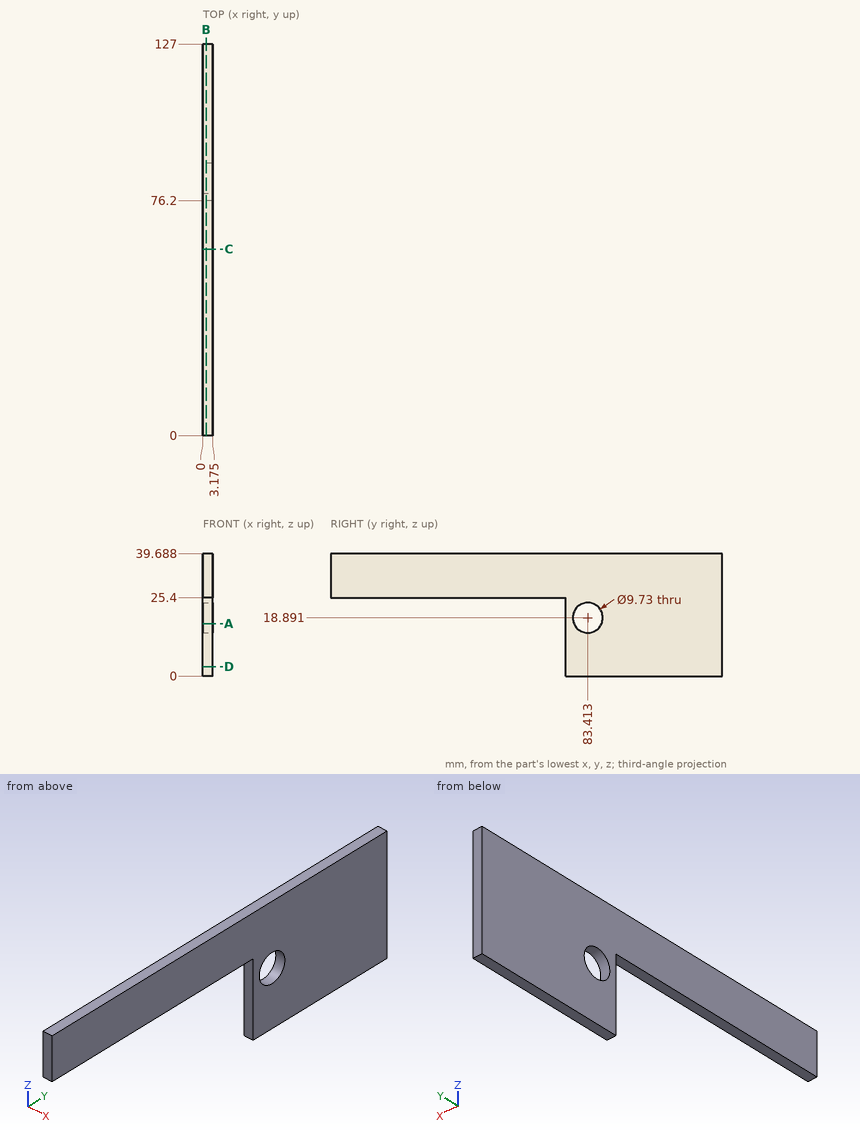
Here's the drawing with two shaded views (mm, measured from the low corner). I have some questions. Coordinates: 2 decimals unless noted, no trailing zeros. Loops run counter-clockwise (first coordinate to the right, second up) from the corner with the lowest first, then second, coordinate; pieces in that order, holes last. Notation, with made-up numbers: (22.25, -7.75) -> (77.25, -7.75) arc R17 cw to (77.25, 4.25) -> close; hole circle Ø7 at (56, 21). An arc over 180 degrees is marked (long way). Answer in a Markdown table with one row per item.
(1) Imagine slicing it at A-A (z = 17). List the corners of the cut face in (x, y) for me (1 decimal), plus the area to 3 significant figures.
Results found:
| item | result |
|---|---|
| outline | (0, 76.2) -> (3.2, 76.2) -> (3.2, 78.9) -> (0, 78.9) -> close; (0, 87.9) -> (3.2, 87.9) -> (3.2, 127) -> (0, 127) -> close |
| area | 133 mm^2 |
(2) Imagine slicing it at C-C (y = 60.5). List the corners of the cut face in (x, z) for me (1 decimal).
Results found:
| item | result |
|---|---|
| outline | (0, 25.4) -> (3.2, 25.4) -> (3.2, 39.7) -> (0, 39.7) -> close |
(3) Imagine slicing it at D-D (z = 3). List the corners of the cut face in (x, y) for me (1 decimal), plus the area to 3 significant figures.
Results found:
| item | result |
|---|---|
| outline | (0, 76.2) -> (3.2, 76.2) -> (3.2, 127) -> (0, 127) -> close |
| area | 161 mm^2 |
(4) If I drill on probe 1 along Y at (x, z) = (2.8, 15.5) (1 decimal); probe 2 along Z at (x, y) = (1, 66.5); probe 3 along Y at (x, z) = (0.9, 9), over which ranges is the centre line in solid material (lowest first)?
Results found:
| item | result |
|---|---|
| probe 1 | y = 76.2 to 79.9, 86.9 to 127 |
| probe 2 | z = 25.4 to 39.69 |
| probe 3 | y = 76.2 to 127 |
(5) Imagine slicing it at B-B (x = 1.1). List the corners of the cut face in (y, z) for me (1 decimal), plus the area to 3 significant figures.
Results found:
| item | result |
|---|---|
| outline | (0, 25.4) -> (76.2, 25.4) -> (76.2, 0) -> (127, 0) -> (127, 39.7) -> (0, 39.7) -> close; hole circle Ø9.7 at (83.4, 18.9) |
| area | 3,030 mm^2 |
(6) Will this pin go through, and if not, where does the flat tip stop? pin 1 Ø1 at (x, y) = (1.5, 35) entering from -Z.
Results found:
| item | result |
|---|---|
| pin 1 | stops at z = 25.4 |
